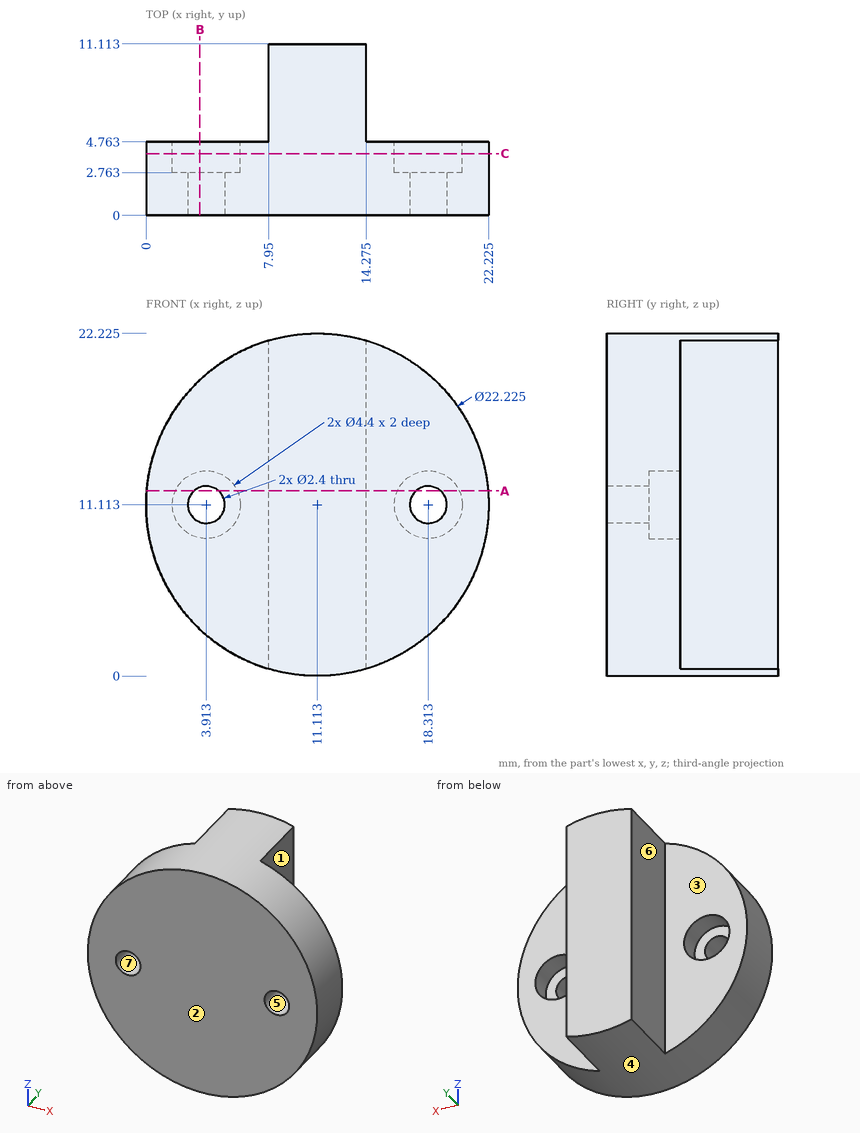
Input: dimensioned drawing with shaded views. Units: mm. Origin: part minimum x, y, z. A direction names the side the tool comes from. Round coordinates to 2 decimals unless told otherwise and drop trailing zeros. Order: outer loops, then holes, each group sorted by start corner. A loop starts at its lowest first (then second) coordinate and runs counter-clockwise, first axis right, second up. Notation, with made-up numbers: (9, 17) -> (29, 17) arc R21 cw to (29, 52) -> close; hole circle Ø5 at (13.25, -35.75). An arc over 180 degrees is marked (long way). One line per item, written item: value. Start each with the question number.
Q1. Access query for the marked faces 1, 2 and 3. Directions: +Z, -Z, +X, -X, +Y, -Y. A direction counts if a zero-diameter tool reaches every point of the face in a straight line with its end or side. Return the directions, or none.
Q2. Draft query along X for the marked faces 4, 5, 6 and 7. Return one class per face: pulls with the +X half, pulls with the -X half, needs draft (parallel to the pull), parting line crosses it, or undercut.
Q3. Section query B-B (x = 3.5). Return the cut outline in (y, z) (1 decimal).
Q4. Section query A-A (z = 12). Give the number of separate pieces and of enclosed holes in the cut face, plus the area to 3 significant figures.
Q5. Material intervals for probe 1 along X at (y, z) = (1.5, 10.75) (1 decimal); probe 2 along Y at (x, z) = (16.75, 11.5); probe 3 along Y at (x, z) = (2.25, 17.5), sorted ascending.
Q6. Pin query (flat end, axial travel): pin 1 (5.5 mm diameter, centred on x = 18.31, z = 11.11, fed in from +Y); pin 2 (3 mm diameter, centred on y = 8, z = 14, fed in from +X) (1 decimal); pin 3 (3 mm diameter, centred on y = 7, z = 9.5, fed in from -X). Return the tip coordinate at first contact, or that it passes through.
Q7. Section query C-C (y = 4). Return the cut outline in (x, z) (1 decimal).
Findings below:
1. face 1: +Z, -Z, +X, +Y
1. face 2: +Z, -Z, +X, -X, -Y
1. face 3: +Z, -Z, -X, +Y
2. face 4: parting line crosses it
2. face 5: undercut
2. face 6: pulls with the -X half
2. face 7: undercut
3. outline: (0, 3) -> (4.8, 3) -> (4.8, 9) -> (2.8, 9) -> (2.8, 10) -> (0, 10) -> close; (0, 12.2) -> (2.8, 12.2) -> (2.8, 13.3) -> (4.8, 13.3) -> (4.8, 19.2) -> (0, 19.2) -> close
4. separate pieces: 3
4. enclosed holes: 0
4. area: 121 mm²
5. probe 1: 0 to 2.8, 5.1 to 17.2, 19.5 to 22.2
5. probe 2: 0 to 2.76
5. probe 3: 0 to 4.76
6. pin 1: y = 4.76
6. pin 2: x = 14.3
6. pin 3: x = 7.95
7. outline: circle Ø22.2 at (11.1, 11.1); hole circle Ø4.4 at (3.9, 11.1); hole circle Ø4.4 at (18.3, 11.1)
